from build123d import *

# Parameters (mm, degrees)
SKETCH1_W           = 5
SKETCH1_H           = 5
BOSS_EXTRUDE1_DEPTH = 74.08
SKETCH2_R           = 1.4
CUT_EXTRUDE1_DEPTH  = 10
SKETCH3_W           = 5
SKETCH3_H           = 5
BOSS_EXTRUDE2_DEPTH = 11.28
SKETCH4_R           = 1.4
CUT_EXTRUDE2_DEPTH  = 10
SKETCH5_R           = 2.5
SKETCH5_R_2         = 1.1
BOSS_EXTRUDE3_DEPTH = 3
FILLET1_R           = 2
SKETCH7_W           = 5
SKETCH7_H           = 3
BOSS_EXTRUDE4_DEPTH = 20.8


with BuildPart() as part:
    # Sketch1 → Boss-Extrude1 (new body)
    with BuildSketch(Plane.XY):
        Rectangle(SKETCH1_W, SKETCH1_H)
    extrude(amount=BOSS_EXTRUDE1_DEPTH)

    # Sketch2 → Cut-Extrude1 (cut)
    with BuildSketch(Plane.XY.offset(74.08)):
        Circle(SKETCH2_R)
    extrude(amount=-CUT_EXTRUDE1_DEPTH, mode=Mode.SUBTRACT)

    # Sketch3 → Boss-Extrude2 (add)
    with BuildSketch(Plane(origin=(2.5, 0, 0), x_dir=(0, 0, -1), z_dir=(1, 0, 0))):
        with Locations((-2.5, 0)):
            Rectangle(SKETCH3_W, SKETCH3_H)
    extrude(amount=BOSS_EXTRUDE2_DEPTH)

    # Sketch4 → Cut-Extrude2 (cut)
    with BuildSketch(Plane(origin=(13.78, 0, 0), x_dir=(0, 0, -1), z_dir=(1, 0, 0))):
        with Locations(Location((-2.5, 0, 0), (0, 0, 90))):
            Circle(SKETCH4_R)
    extrude(amount=-CUT_EXTRUDE2_DEPTH, mode=Mode.SUBTRACT)

    # Sketch5 → Boss-Extrude3 (add)
    # profile 1 of 2: a face of its own
    with BuildSketch(Plane(origin=(0, 2.5, 0), x_dir=(1, 0, 0), z_dir=(0, 1, 0))):
        with Locations(Location((0, -60.5, 0), (0, 0, 180))):
            Circle(SKETCH5_R)
        with Locations(Location((0, -60.5, 0), (0, 0, 270))):
            Circle(SKETCH5_R_2, mode=Mode.SUBTRACT)
    # profile 2 of 2: a face of its own
    with BuildSketch(Plane(origin=(0, 2.5, 0), x_dir=(1, 0, 0), z_dir=(0, 1, 0))):
        with Locations(Location((0, -2.5, 0), (0, 0, 90))):
            Circle(SKETCH5_R)
        with Locations(Location((0, -2.5, 0), (0, 0, 270))):
            Circle(SKETCH5_R_2, mode=Mode.SUBTRACT)
    extrude(amount=BOSS_EXTRUDE3_DEPTH)

    # Fillet1
    fillet1_edges = [part.edges().sort_by_distance(p)[0] for p in [
        (2.5, 0, 5),
        (-2.5, 0, 0),
    ]]
    fillet(fillet1_edges, radius=FILLET1_R)

    # Sketch7 → Boss-Extrude4 (add)
    with BuildSketch(Plane(origin=(0, 2.5, 0), x_dir=(1, 0, 0), z_dir=(0, 1, 0))):
        with Locations((0, -66.5)):
            Rectangle(SKETCH7_W, SKETCH7_H)
    extrude(amount=BOSS_EXTRUDE4_DEPTH)


solid = part.part
Build history of the part. All positions in model axes, mm. A direction names the side the tool comes from. Coordinates: 2 decimals unless noted, no trailing zeros. Write each loop counter-clockwise with the first axis right and the second up, starting at its lowest first coordinate (ties: lowest second). Pieces come first, ordered by that corner, then holes. Notation, with made-up numbers: (-3, 19) -> (49, 19) arc R26 cw to (49, 42) -> close; hole circle Ø9 at (-0.5, 31). An arc over 180 degrees is marked (long way). Use CSV: the item, a comma, the result in double quotes. Start each with the question number.
Q1. Cut at C-C, the plane z = 48. List the corners of the cut face in (x, y).
Q2. Pull direction X, two halves, no side cores. Call faces 5 (the flat face through (0, 13, 68)), 6 (the cylindrical face through (0, 4, 59.4)), 7 (the flat face through (2.5, 2, 48)): released by +X, released by -X, zero draft, split by the parting line, or undercut.
Q3. Flat gauge pins, fed straight in: pin 1 Ø2 at (x, y) = (1, 7) entering from +Z; pin 2 Ø2.5 at (x, y) = (8.5, 1) entering from +Z; pin 3 Ø1 at (y, z) = (3.5, 53) entering from -X; pin 4 Ø5.5 at (x, z) = (1, 60) entering from +Y. Where does each tip first touch, or does it go through?
Q4. Drill centre lines: probe 1 along X at (y, z) = (3.2, 2.5); probe 2 along X at (y, z) = (-0.75, 42). Where is each one in solid material? Low to high.
Q5. Cut at A-A, the plane y = 0. List the corners of the cut face in (x, z).
Q6. 3-axis set-ups, long thin cutter, end or side, ignore diameter. For faces 1 (the cylindrical face through (8.85, -0.303, 1.133)), 2 (the flat face through (9, 0, 5)), 3 (the cylindrical face through (0.54, 3.98, 58.06)), 4 (the flat face through (0, 0, 64.08)): which of +Z, -Z, +X, -X, +Y, -Y reach the whole face in a straight line?
Q7. Cut at B-B, the plane x = 5.5. List the corners of the cut face in (y, z).
Q8. Cut at D-D, the plane y = 16.5. List the corners of the cut face in (x, z).
Checked values:
1,outline,"(-2.5, -2.5) -> (2.5, -2.5) -> (2.5, 2.5) -> (-2.5, 2.5) -> close"
2,face 5,"zero draft"
2,face 6,"undercut"
2,face 7,"released by +X"
3,pin 1,"stops at z = 68"
3,pin 2,"stops at z = 5"
3,pin 3,"passes through"
3,pin 4,"stops at y = 5.5"
4,probe 1,"x = -2.5 to -1.1, 1.1 to 2.5"
4,probe 2,"x = -2.5 to 2.5"
5,outline,"(-2.5, 2) arc R2 ccw to (-0.5, 0) -> (13.78, 0) -> (13.78, 1.1) -> (3.78, 1.1) -> (3.78, 3.9) -> (13.78, 3.9) -> (13.78, 5) -> (4.5, 5) arc R2 cw to (2.5, 7) -> (2.5, 74.08) -> (1.4, 74.08) -> (1.4, 64.08) -> (-1.4, 64.08) -> (-1.4, 74.08) -> (-2.5, 74.08) -> close"
6,face 1,"+X"
6,face 2,"+Z, +X, +Y, -Y"
6,face 3,"+Y"
6,face 4,"+Z"
7,outline,"(-2.5, 0) -> (2.5, 0) -> (2.5, 5) -> (-2.5, 5) -> close; hole circle Ø2.8 at (0, 2.5)"
8,outline,"(-2.5, 65) -> (2.5, 65) -> (2.5, 68) -> (-2.5, 68) -> close"
